The listing builds one solid part. Answer for the finished solid, in the listing's coordinates (mm). A direction names the side the tool comes from. Round coordinates to 2 decimals unless told otherwise and drop trailing zeros. Loops run counter-clockwise (first coordinate to the right, second up) from the corner with the lowest first, then second, coordinate; pieces in that order, holes last. Notation, with made-up numbers: M 35,52 L 63,52 A26 cw 63,73 Z; hole C 88.25,31.5 d5. An arc over 180 degrees is marked long. Answer as a JSON object with one key per item and string values.
Autodesk Inventor part; units mm, degrees
ref_plane "YZ Plane" through (0, 0, 0) normal (1, 0, 0) x (0, 1, 0)
ref_plane "XZ Plane" through (0, 0, 0) normal (0, 1, 0) x (-1, 0, 0)
ref_plane "XY Plane" through (0, 0, 0) normal (0, 0, 1) x (1, 0, 0)
sketch "Sketch1" plane through (0, 0, 0) normal (0, 0, 1) x (1, 0, 0)
  line L0 (-8.89, 0) -> (8.89, 0) construction
  line L1 (0, -8.05) -> (0, 8.05) construction
  line L2 (-6.35, 5.75) -> (6.35, 5.75)
  line L3 (6.35, 5.75) -> (6.35, -5.75)
  line L4 (6.35, -5.75) -> (-6.35, -5.75)
  line L5 (-6.35, -5.75) -> (-6.35, 5.75)
  point P0 (0, 0)
  point P1 (0, 5.75)
  point P2 (6.35, 0)
  dimension "d0" = 12.7
  dimension "d1" = 11.5
extrude "Extrusion1" add sketch "Sketch1" along normal blind 9.5
sketch "Sketch2" plane through (0, 0, 9.5) normal (0, 0, 1) x (1, 0, 0)
  circle A0 centre (0, 0) radius 4
  dimension "d4" = 8
extrude "Extrusion2" add sketch "Sketch2" along normal blind 1
sketch "Sketch3" plane through (0, 0, 10.5) normal (0, 0, 1) x (1, 0, 0)
  circle A0 centre (0, 0) radius 3.1
  dimension "d7" = 6.2
extrude "Extrusion3" add sketch "Sketch3" along normal blind 7.5
sketch "Sketch4" plane through (0, 0, 0) normal (0, 1, 0) x (-1, 0, 0)
  line L0 (8.89, 0) -> (-8.89, 0) construction
  line L1 (0, -3.6) -> (0, 21.6) construction
  line L2 (0, 13) -> (-4.5899, 30.1296) construction
  line L3 (3.1, 18) -> (-3.1, 18) construction
  line L4 (-1.2212, 17.5575) -> (-2.4088, 17.2393)
  line L5 (-2.4088, 17.2393) -> (-5.3768, 27.271)
  line L6 (-5.3768, 27.271) -> (-3.9279, 27.6593)
  line L7 (-3.9279, 27.6593) -> (-1.2212, 17.5575)
  point P0 (0, 0)
  point P1 (-1.3397, 18)
  point P2 (-2.6338, 18)
  dimension "d10" = 15
  dimension "d11" = 5
  dimension "d13" = 10
  dimension "d14" = 3
  dimension "d16" = 2.5
revolve "Revolution1" add sketch "Sketch4" angle 360 about axis through (0, 0, 13) along (0.258819, 0, 0.9659258)
fillet "Fillet1" radius 1.4 1 edges at (2.479, 0, 28.0475)
properties part number "F112"
Item 1: The part is cut by section B-B (y = 5). Give the vertices of the cut face in (x, z).
Values follow:
{"outline": "M -6.35,0 L 6.35,0 L 6.35,9.5 L -6.35,9.5 Z"}
Item 2: The part is cut by section A-A (x = -1.75). Give the vertices of the cut face in (y, z).
Values follow:
{"outline": "M -5.75,0 L 5.75,0 L 5.75,9.5 L 3.6,9.5 L 3.6,10.5 L 2.56,10.5 L 2.56,18 L -2.56,18 L -2.56,10.5 L -3.6,10.5 L -3.6,9.5 L -5.75,9.5 Z"}
Item 3: Determine the mould class of faces 3 (the face through (0, -5.75, 5)), 4 (the face through (1.119, 0.059, 22.383)), 5 (the face through (2, -3, 10.5)), 6 (the face through (0, 0, 0)) for opening direction Z: released by +Z, released by -Z, zero draft, split by the parting line, or undercut.
Values follow:
{"face 3": "zero draft", "face 4": "undercut", "face 5": "undercut", "face 6": "released by -Z"}
Item 4: Straight lines are drawn through the part: line 1 (Z direction, x = 3.25, y = -2.75); line 2 (Z direction, x = -1.5, y = -3); line 3 (Y direction, x = 0, z = 15.5). For each, find the intervals that lie inside material, in ascending order.
Values follow:
{"line 1": "0 to 9.5", "line 2": "0 to 10.5", "line 3": "-3.1 to 3.1"}
Item 5: Flat-ended cylindrical pins translate along their axes: P1, Ø5, axis at x = 4.5, z = 15, coming from the -Y side; P2, Ø4, axis at x = -4.5, y = 1.5, coming from the +Z side; P3, Ø6, axis at y = 1, z = 24, coming from the +X side. Find the tip coordinate at first contact, or state that the pin passes through.
Values follow:
{"P1": "y = -2.37", "P2": "z = 18", "P3": "x = 5.03"}
Item 6: Which of the six approach directions +Z, -Z, +X, -X, +Y, -Y give full straight-line access (tool end or side, diameter ignored) to faces 1 (the face through (-6.35, 0, 5)), 2 (the face through (1.43, 2.75, 14.2))?
Values follow:
{"face 1": "+Z, -Z, -X, +Y, -Y", "face 2": "none"}
